The listing builds one solid part. Answer for the finished solid, in the listing's coordinates (mm). Face numbers are marked on the shaded views. A direction names the side the tool comes from. Coordinates: 2 decimals unless noted, no trailing zeros. Order: outer loops, then holes, each group sorted by start corner. A loop starts at its lowest first (then second) coordinate and runs counter-clockwise, first axis right, second up. Notation, with made-up numbers: (-37, 89) -> (8, 89) arc R30 ccw to (8, 116) -> close; hole circle Ø9 at (81, 46). An arc over 180 degrees is marked (long way). Write item = value, one per line.
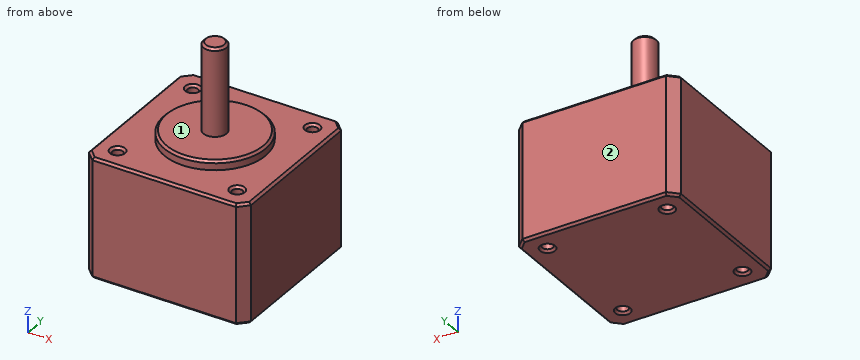
from build123d import *

# Parameters (mm, degrees)
F0_W     = 35.2
F0_H     = 35.2
F4_DEPTH = 26
F1_R     = 11
F5_DEPTH = 2
F2_R     = 2.5
F6_DEPTH = 21
F3_R     = 1.15
F7_DEPTH = 26.001
F8_SIZE  = 2
F9_SIZE  = 0.5


with BuildPart() as f4:
    # F0 (on Top) → F4 (new body)
    with BuildSketch(Plane.XY):
        Rectangle(F0_W, F0_H)
    extrude(amount=-F4_DEPTH)

    # F1 (on Top) → F5 (join)
    with BuildSketch(Plane.XY):
        Circle(F1_R)
    extrude(amount=F5_DEPTH)

    # F2 (on Top) → F6 (join)
    with BuildSketch(Plane.XY):
        Circle(F2_R)
    extrude(amount=F6_DEPTH)

    # F3 (on Top) → F7 (cut, through all)
    with BuildSketch(Plane.XY):
        with Locations((-13, -13)):
            Circle(F3_R)
        with Locations((13, -13)):
            Circle(F3_R)
        with Locations((13, 13)):
            Circle(F3_R)
        with Locations((-13, 13)):
            Circle(F3_R)
    extrude(amount=-F7_DEPTH, mode=Mode.SUBTRACT)

    # F8
    f8_edges = [f4.edges().sort_by_distance(p)[0] for p in [
        (17.6, -17.6, -13),
        (-17.6, -17.6, -13),
        (-17.6, 17.6, -13),
        (17.6, 17.6, -13),
    ]]
    chamfer(f8_edges, length=F8_SIZE)

    # F9
    f9_edges = [f4.edges().sort_by_distance(p)[0] for p in [
        (-2.5, 0, 21),
        (-11, 0, 2),
        (11.85, 13, 0),
        (11.85, -13, 0),
        (-14.15, -13, 0),
        (-14.15, 13, 0),
        (0, 17.6, 0),
        (16.6, 16.6, 0),
        (17.6, 0, 0),
        (16.6, -16.6, 0),
        (0, -17.6, 0),
        (-17.6, 0, 0),
        (17.6, 0, -26),
        (0, -17.6, -26),
        (11.85, -13, -26),
        (16.6, -16.6, -26),
        (-14.15, -13, -26),
        (11.85, 13, -26),
        (-14.15, 13, -26),
        (0, 17.6, -26),
        (-16.6, 16.6, -26),
        (16.6, 16.6, -26),
        (-17.6, 0, -26),
        (-16.6, -16.6, -26),
        (-16.6, 16.6, 0),
        (-16.6, -16.6, 0),
    ]]
    chamfer(f9_edges, length=F9_SIZE)


solid = f4.part
Q1. A tool of negligible diameter and unlimited length cuts with its end or side. For the marked faces 1 and 2, from which of +Z, -Z, +X, -X, +Y, -Y can it reach the whole face along a straight path? Write none if from no direction.
The answers:
face_1 = +Z
face_2 = +Z, -Z, +X, -X, +Y
Q2. Section A-A, the plane y = 13 is taken. Give the vertices of the cut face in (x, z), plus the area to 3 significant figures.
The answers:
outline = (-17.6, -25.5) -> (-17.1, -26) -> (-14.65, -26) -> (-14.15, -25.5) -> (-14.15, -0.5) -> (-14.65, 0) -> (-17.1, 0) -> (-17.6, -0.5) -> close; (-11.85, -25.5) -> (-11.35, -26) -> (11.35, -26) -> (11.85, -25.5) -> (11.85, -0.5) -> (11.35, 0) -> (-11.35, 0) -> (-11.85, -0.5) -> close; (14.15, -25.5) -> (14.65, -26) -> (17.1, -26) -> (17.6, -25.5) -> (17.6, -0.5) -> (17.1, 0) -> (14.65, 0) -> (14.15, -0.5) -> close
area = 794 mm2
Q3. Section C-C, the plane x = 0 is taken. Give the vertices of the cut face in (y, z), plus the area to 3 significant figures.
The answers:
outline = (-17.6, -25.5) -> (-17.1, -26) -> (17.1, -26) -> (17.6, -25.5) -> (17.6, -0.5) -> (17.1, 0) -> (11, 0) -> (11, 1.5) -> (10.5, 2) -> (2.5, 2) -> (2.5, 20.5) -> (2, 21) -> (-2, 21) -> (-2.5, 20.5) -> (-2.5, 2) -> (-10.5, 2) -> (-11, 1.5) -> (-11, 0) -> (-17.1, 0) -> (-17.6, -0.5) -> close
area = 1,050 mm2
Q4. Find the intervals of material crossed by line 1 along Y through (x, z) = (-13, -9.25); line 2 along Z through (x, y) = (7.5, -10); line 3 along Y through (x, z) = (-13.5, -24), in increasing order.
The answers:
line_1 = -17.6 to -14.15, -11.85 to 11.85, 14.15 to 17.6
line_2 = -26 to 0
line_3 = -17.6 to -14.04, -11.96 to 11.96, 14.04 to 17.6
Q5. This flat-tipped pin is pushed along its axis until it touches: pin 1 Ø2.5 at (x, y) = (-13, 13) entering from +Z. Where does it stop, or does it pass through?
The answers:
pin_1 = -0.4
Q6. Section B-B, the plane z = -21.5 is taken. Give the vertices of the cut face in (x, y).
The answers:
outline = (-17.6, -15.6) -> (-15.6, -17.6) -> (15.6, -17.6) -> (17.6, -15.6) -> (17.6, 15.6) -> (15.6, 17.6) -> (-15.6, 17.6) -> (-17.6, 15.6) -> close; hole circle Ø2.3 at (-13, -13); hole circle Ø2.3 at (-13, 13); hole circle Ø2.3 at (13, -13); hole circle Ø2.3 at (13, 13)
